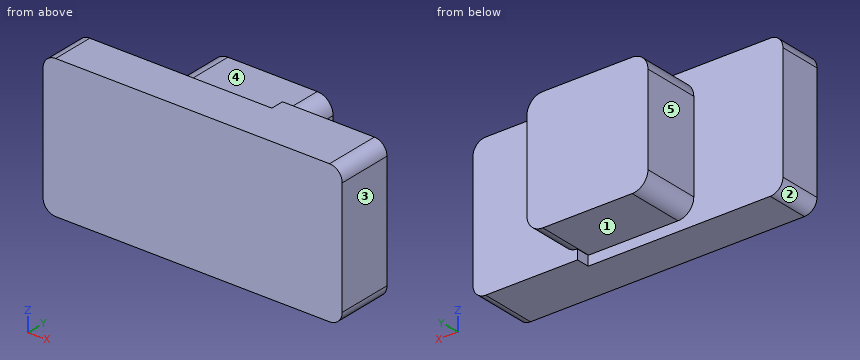
from build123d import *

# Parameters (mm, degrees)
BOSS_EXTRUDE1_DEPTH = 44.3
SKETCH2_W           = 38.2
SKETCH2_H           = 38.2
BOSS_EXTRUDE2_DEPTH = 18.02
FILLET1_R           = 5
FILLET2_R           = 4


with BuildPart() as part:
    # Sketch1 → Boss-Extrude1 (new body)
    with BuildSketch(Plane.XY):
        Polygon((0, 0), (-77.858285242, 0), (-77.858285242, 13.4), (-16.398285242, 13.4), (-16.398285242, 17.6), (16.601714758, 17.6), (16.601714758, 0), align=None)
    extrude(amount=BOSS_EXTRUDE1_DEPTH)

    # Sketch2 → Boss-Extrude2 (add)
    with BuildSketch(Plane(origin=(0, 13.4, 0), x_dir=(1, 0, 0), z_dir=(0, 1, 0))):
        with Locations((-30.628285242, -22.15)):
            Rectangle(SKETCH2_W, SKETCH2_H)
    extrude(amount=BOSS_EXTRUDE2_DEPTH)

    # Fillet1
    fillet1_edges = [part.edges().sort_by_distance(p)[0] for p in [
        (-49.728285242, 22.41, 3.05),
        (-11.528285242, 24.51, 3.05),
        (-11.528285242, 24.51, 41.25),
        (-49.728285242, 22.41, 41.25),
    ]]
    fillet(fillet1_edges, radius=FILLET1_R)

    # Fillet2
    fillet2_edges = [part.edges().sort_by_distance(p)[0] for p in [
        (-77.858285242, 6.7, 44.3),
        (-77.858285242, 6.7, 0),
        (16.601714758, 8.8, 44.3),
        (16.601714758, 8.8, 0),
    ]]
    fillet(fillet2_edges, radius=FILLET2_R)


solid = part.part
Source: CAD feature listing. Evaluate the final solid. Frame: model axes, mm. Face numbers are marked on the shaded views. A direction names the side the tool comes from. Give positions to 0.01 mm unless a question says otherwise; leave off trailing zeros. Order: outer loops, then holes, each group sorted by start corner. A loop starts at its lowest first (then second) coordinate and runs counter-clockwise, first axis right, second up. Notation, with made-up numbers: (7.25, -29.5) -> (12.25, -29.5) arc R11 cw to (12.25, -11.5) -> close; hole circle Ø7 at (-10, 83.5). An arc over 180 degrees is marked (long way). Use a Markdown table: item, result.
1) Section query C-C, the plane x = -58. Return the cut outline in (y, z), then the cut area to 3 significant figures.
Answer list:
| item | result |
|---|---|
| outline | (0, 0) -> (13.4, 0) -> (13.4, 44.3) -> (0, 44.3) -> close |
| area | 594 mm² |
2) Section query D-D, the plane x = 9. Return the cut outline in (y, z), then the cut area to 3 significant figures.
Answer list:
| item | result |
|---|---|
| outline | (0, 0) -> (17.6, 0) -> (17.6, 44.3) -> (0, 44.3) -> close |
| area | 780 mm² |
3) Contact query for flat-ended pins moving along their axis: P1, Ø5.5, axis at x = -24.5, y = 18, coming from the +Z side; P2, Ø13.5, axis at x = -62, z = 19, coming from the +Y side; P3, Ø0.9, axis at y = 16, z = 1.5, coming from the -X side. Output: stop coordinate, or through.
Answer list:
| item | result |
|---|---|
| P1 | z = 41.25 |
| P2 | y = 13.4 |
| P3 | x = -16.4 |
4) Reachability of the marked faces 1, 2, 3, 4 and 5 from +Z, -Z, +X, -X, +Y, -Y: full face, straight path, thin tool, end or side. Return the list, or none.
Answer list:
| item | result |
|---|---|
| face 1 | -Z, -X, +Y |
| face 2 | -Z, -X, +Y, -Y |
| face 3 | +Z, -Z, +X, +Y, -Y |
| face 4 | +Z, -X, +Y |
| face 5 | +Z, -Z, -X, +Y |
5) Section query A-A, the plane y = 29. Return the cut outline in (x, z).
Answer list:
| item | result |
|---|---|
| outline | (-49.73, 8.05) arc R5 ccw to (-44.73, 3.05) -> (-16.53, 3.05) arc R5 ccw to (-11.53, 8.05) -> (-11.53, 36.25) arc R5 ccw to (-16.53, 41.25) -> (-44.73, 41.25) arc R5 ccw to (-49.73, 36.25) -> close |
6) Ray query, line 1 along X through (y, z) = (24, 16.5); line 2 along Y through (x, z) = (13, 37.5); line 3 along Y through (x, z) = (-70.5, 4). Return the intervals inside material, ascending. Write a range as [from, to].
Answer list:
| item | result |
|---|---|
| line 1 | [-49.73, -11.53] |
| line 2 | [0, 17.6] |
| line 3 | [0, 13.4] |
7) Section query B-B, the plane z = 19.5. Return the cut outline in (x, y).
Answer list:
| item | result |
|---|---|
| outline | (-77.86, 0) -> (16.6, 0) -> (16.6, 17.6) -> (-11.53, 17.6) -> (-11.53, 31.42) -> (-49.73, 31.42) -> (-49.73, 13.4) -> (-77.86, 13.4) -> close |
